from build123d import *

# Parameters (mm, degrees)
F1_DEPTH = 1.5
F2_W     = 21.121388
F2_H     = 49.146654
F2_W_2   = 9.488664
F2_H_2   = 11.803286
F2_W_3   = 9.919964
F2_W_4   = 9.919956
F3_DEPTH = 1.5


with BuildPart() as f1:
    # F0 (on Right) → F1 (new body)
    with BuildSketch(Plane.YZ):
        Polygon((-80.233574, -9.394377), (-80.233574, -33.967704), (90.941433, -33.967704), (145.892367, 14.248275), (102.09786, 27.465614), (-48.834328, 27.465614), align=None)
    extrude(amount=F1_DEPTH)

    # F2 (on face) → F3 (cut)
    with BuildSketch(Plane.YZ.offset(1.5)):
        Polygon((-50.199509, 18.364381), (-70.904814, -6.436477), (-45.421362, -6.436477), (-45.421362, 18.364381), align=None)
        with Locations((-20.753761, -6.208946)):
            Rectangle(F2_W, F2_H)
        with Locations((19.782484, 12.462738)):
            Rectangle(F2_W_2, F2_H_2)
        with Locations((40.053718, 12.462738)):
            Rectangle(F2_W_3, F2_H_2)
        with Locations((59.46235, 12.462738)):
            Rectangle(F2_W_2, F2_H_2)
        with Locations((80.596194, 12.462738)):
            Rectangle(F2_W_4, F2_H_2)
    extrude(amount=-F3_DEPTH, mode=Mode.SUBTRACT)


solid = f1.part
Build history of the part. All positions in model axes, mm. Give positions to 0.01 mm unless a question says otherwise; leave off trailing zeros. Order: outer loops, then holes, each group sorted by start corner. A loop starts at its lowest first (then second) coordinate and runs counter-clockwise, first axis right, second up. Notation, with made-up numbers: M 88.5,45.25 L 137.5,45.25 A31 cw 137.5,71.25 Z; hole C 77,-9.75 d3. An arc over 180 degrees is marked long. Put each result on its own line as item: value.
Item 1: Drop flat-ended pins along their axis: pin 1 Ø0.8 at (x, z) = (1, -17.5) entering from +Y; pin 2 Ø0.8 at (x, z) = (1, 14.5) entering from -Y. Give the stop position or say it passes through.
Results are:
pin 1: y = 110.17
pin 2: y = -60.22
Item 2: Pull direction Y, two halves, no side cores. Call faces 1 (the face through (0.74, 124.302, 20.764)), 2 (the face through (1.5, 31, -3)), 3 (the face through (0.76, -60.407, 6.138)), 4 (the face through (0.74, -64.314, 9.294)): +Y half, -Y half, draft (parallel to the pull), parting line (faces both ways), or undercut.
Results are:
face 1: +Y half
face 2: draft
face 3: undercut
face 4: -Y half
Item 3: Cut at C-C on x = 0.7. Count the separate pieces of the cut face and the enclosed holes in it, then the cut area to 3 significant figures.
Results are:
separate pieces: 1
enclosed holes: 6
area: 9,830 mm2
Item 4: Cut at D-D on z = -1. Write the cut outline in (x, y).
Results are:
outline: M 0,-73.08 L 1.5,-73.08 L 1.5,-66.37 L 0,-66.37 Z; M 0,-45.42 L 1.5,-45.42 L 1.5,-31.31 L 0,-31.31 Z; M 0,-10.19 L 1.5,-10.19 L 1.5,128.51 L 0,128.51 Z
Item 5: Wall check: probe 1 along Z at (x, y) = (1, -18); probe 2 along Z at (x, y) = (0.85, 22.5); probe 3 along Y at (x, z) = (0.6, -5.5). Give the ranges that are in metal, low to high.
Results are:
probe 1: -33.97 to -30.78, 18.36 to 27.47
probe 2: -33.97 to 6.56, 18.36 to 27.47
probe 3: -76.92 to -70.12, -45.42 to -31.31, -10.19 to 123.39
Item 6: Cut at B-B on z = -22.5. Write the cut outline in (x, y).
Results are:
outline: M 0,-80.23 L 1.5,-80.23 L 1.5,-31.31 L 0,-31.31 Z; M 0,-10.19 L 1.5,-10.19 L 1.5,104.01 L 0,104.01 Z
Item 7: Cut at A-A on y = 21.5. Write the cut outline in (x, z).
Results are:
outline: M 0,-33.97 L 1.5,-33.97 L 1.5,6.56 L 0,6.56 Z; M 0,18.36 L 1.5,18.36 L 1.5,27.47 L 0,27.47 Z
